from build123d import *

# Parameters (mm, degrees)
SKETCH_1_R          = 2.1
EXTRUDE_1_DEPTH     = 6
EXTRUDE_START       = -6
SKETCH_2_W          = 102
SKETCH_2_H          = 39
SKETCH_2_R          = 2.1
EXTRUDE_2_DEPTH     = 6
CUT_EXTRUDE_START   = -3
SKETCH_3_R          = 2.1
CUT_EXTRUDE_2_DEPTH = 3
FILLET_1_R          = 3


with BuildPart() as part:
    # 草图1 → 凸台-拉伸1 (new body)
    with BuildSketch(Plane.XY):
        Polygon((-42.425, -5), (42.425, -5), (3.425, 34), (-3.425, 34), align=None)
        with Locations((0, 30)):
            Circle(SKETCH_1_R, mode=Mode.SUBTRACT)
        with Locations((-32, 0)):
            Circle(SKETCH_1_R, mode=Mode.SUBTRACT)
        with Locations((32, 0)):
            Circle(SKETCH_1_R, mode=Mode.SUBTRACT)
    extrude(amount=EXTRUDE_1_DEPTH)

    # 草图2 → 凸台-拉伸2 (add)
    with BuildSketch(Plane.XY.offset(6).offset(EXTRUDE_START)):
        with Locations((0, 14.5)):
            Rectangle(SKETCH_2_W, SKETCH_2_H)
        with Locations((-46, -0.5)):
            Circle(SKETCH_2_R, mode=Mode.SUBTRACT)
        with Locations((-46, 29.5)):
            Circle(SKETCH_2_R, mode=Mode.SUBTRACT)
        with Locations((46, 29.5)):
            Circle(SKETCH_2_R, mode=Mode.SUBTRACT)
        with Locations((46, -0.5)):
            Circle(SKETCH_2_R, mode=Mode.SUBTRACT)
        with Locations((-32, 0)):
            Circle(SKETCH_2_R, mode=Mode.SUBTRACT)
        with Locations((0, 30)):
            Circle(SKETCH_2_R, mode=Mode.SUBTRACT)
        with Locations((32, 0)):
            Circle(SKETCH_2_R, mode=Mode.SUBTRACT)
    extrude(amount=EXTRUDE_2_DEPTH)

    # 草图3 → 切除-拉伸2 (cut)
    with BuildSketch(Plane.XY.offset(6).offset(CUT_EXTRUDE_START)):
        Polygon((-3.425, 34), (-3.566421356, 34), (-42.495710678, -4.929289322), (-42.566421356, -5), (-42.425, -5), (42.425, -5), (42.566421356, -5), (42.495710678, -4.929289322), (3.566421356, 34), (3.425, 34), align=None)
        with Locations((-32, 0)):
            Circle(SKETCH_3_R, mode=Mode.SUBTRACT)
        with Locations((32, 0)):
            Circle(SKETCH_3_R, mode=Mode.SUBTRACT)
        with Locations((0, 30)):
            Circle(SKETCH_3_R, mode=Mode.SUBTRACT)
    extrude(amount=CUT_EXTRUDE_2_DEPTH, mode=Mode.SUBTRACT)

    # 圆角1
    fillet_1_edges = [part.edges().sort_by_distance(p)[0] for p in [
        (-51, 34, 3),
        (51, -5, 3),
        (-51, -5, 3),
        (51, 34, 3),
    ]]
    fillet(fillet_1_edges, radius=FILLET_1_R)


solid = part.part
Can you work these out from the model? Positions are in its coordinate system, mm. A direction names the side the tool comes from. Give positions to 0.01 mm unless a question says otherwise; leave off trailing zeros. Loops run counter-clockwise (first coordinate to the right, second up) from the corner with the lowest first, then second, coordinate; pieces in that order, holes last. Notation, with made-up numbers: M -20.5,45.5 L 24.5,45.5 A21 ccw 24.5,67.5 Z; hole C 37.25,57 d11. An arc over 180 degrees is marked long. One line per item, written item: value. Start each with the question number.
1) If we section it at B-B, the plane x = 46: Write out the boundary of the cut face in (y, z).
2) If we section it at C-C, the plane x = 32: Write out the boundary of the cut face in (y, z), and give its area (3 significant figures).
3) If we section it at A-A, the plane z = 1.65: Write out the boundary of the cut face in (x, y).
4) On a 3-axis mill with a long thin cutter (end or side, diameter ignored), from which of +Z, -Z, +X, -X, +Y, -Y can I reach the whole of each face in a straight line? I mean faces 1 (the face through (-44.06, -1.3, 2.96)), 2 (the face through (-1, 10, 3)). Say none if no direction works.
5) If we section it at D-D, the plane y = 13: Write out the boundary of the cut face in (x, z), and give its area (3 significant figures).
6) Thinking about a two-plate mould opening in X: for faces 3 (the face through (23.339, 14.227, 4.479)), 4 (the face through (-50.14, -4.1, 3.04)), 5 (the face through (-45.031, 27.637, 2.958)), 6 (the face through (-1, 34, 2)), which applies, +X half, -X half, draft (parallel to the pull), parting line (faces both ways), or undercut?
7) If I drill on line 1 (Y direction, x = -46, z = 4.5); line 2 (Y direction, x = -32, z = 1.55); line 3 (X direction, y = -1, z = 0.95), over which ranges is the centre line in solid material (lowest first)? Write a range as [from, to].
8) I'm going to push a flat-ended pin straight in: pin 1 (2.5 mm diameter, centred on x = -46, y = -0.5, fed in from -Z). Where does the tip first touch, or does it pass through?
Completed:
1. outline: M -5,0 L -2.6,0 L -2.6,6 L -5,6 Z; M 1.6,0 L 27.4,0 L 27.4,6 L 1.6,6 Z; M 31.6,0 L 34,0 L 34,6 L 31.6,6 Z
2. outline: M -5,0 L -2.1,0 L -2.1,3 L -5,3 Z; M 2.1,0 L 34,0 L 34,6 L 5.57,6 L 5.57,3 L 2.1,3 Z
2. area: 190 mm^2
3. outline: M -51,-2 A3 ccw -48,-5 L 48,-5 A3 ccw 51,-2 L 51,31 A3 ccw 48,34 L -48,34 A3 ccw -51,31 Z; hole C -46,-0.5 d4.2; hole C -46,29.5 d4.2; hole C -32,0 d4.2; hole C 0,30 d4.2; hole C 32,0 d4.2; hole C 46,-0.5 d4.2; hole C 46,29.5 d4.2
4. face 1: +Z, -Z
4. face 2: +Z, -Y
5. outline: M -51,0 L 51,0 L 51,6 L 24.57,6 L 24.57,3 L -24.57,3 L -24.57,6 L -51,6 Z
5. area: 465 mm^2
6. face 3: undercut
6. face 4: -X half
6. face 5: undercut
6. face 6: draft
7. line 1: y = [-5, -2.6], [1.6, 27.4], [31.6, 34]
7. line 2: y = [-5, -2.1], [2.1, 34]
7. line 3: x = [-51, -48.04], [-43.96, -33.85], [-30.15, 30.15], [33.85, 43.96], [48.04, 51]
8. pin 1: passes through
